Here's how the part is built. I have some questions about the finished solid (model axes, mm). Face numbers are marked on the shaded views. A direction names the side the tool comes from. Coordinates: 2 decimals unless noted, no trailing zeros. Write each loop counter-clockwise with the first axis right and the second up, starting at its lowest first coordinate (ties: lowest second). Pieces come first, ordered by that corner, then holes.
```python
from build123d import *

# Parameters (mm, degrees)
SKETCH1_R              = 2.35
PIN_DEPTH              = 11.35
SKETCH2_R              = 2.95
MIDDLE_DEPTH           = 4.8
SKETCH3_R              = 2.625
OUTER_RIM_DEPTH        = 0.5
BORE_CUT_DEPTH         = 13.562941535
SLOT_CUT_DEPTH         = 13.562941535
SLOT_CUT_DEPTH_BACK    = 13.562941535
SKETCH6_R              = 3.7
MIDDLE_BODY_DEPTH      = 3.9
MIDDLE_BORE_DEPTH      = 14.012398084
MIDDLE_BORE_DEPTH_BACK = 14.012398084
SKETCH7_R              = 2.4
SKETCH8_R              = 3.05
MIDDLE_RIM_CUT_DEPTH   = 0.75


with BuildPart() as part:
    # Sketch1 → Pin (new body)
    with BuildSketch(Plane(origin=(0, 0, 0), x_dir=(0, 0, -1), z_dir=(1, 0, 0))):
        Circle(SKETCH1_R)
    extrude(amount=PIN_DEPTH)

    # Sketch2 → Middle (add)
    with BuildSketch(Plane(origin=(0, 0, 0), x_dir=(0, 0, -1), z_dir=(1, 0, 0))):
        Circle(SKETCH2_R)
    extrude(amount=MIDDLE_DEPTH)

    # Sketch3 → Outer Rim (add)
    with BuildSketch(Plane(origin=(11.35, 0, 0), x_dir=(0, 0, -1), z_dir=(1, 0, 0))):
        Circle(SKETCH3_R)
    extrude(amount=OUTER_RIM_DEPTH)

    # Sketch4 → Bore Cut (cut, through all)
    with BuildSketch(Plane(origin=(0, 0, 0), x_dir=(0, 0, -1), z_dir=(1, 0, 0))):
        with BuildLine():
            ThreePointArc((-1.1, -1.393063172), (0, -1.775), (1.1, -1.393063172))
            Line((1.1, -1.393063172), (1.1, 1.393063172))
            ThreePointArc((1.1, 1.393063172), (0, 1.775), (-1.1, 1.393063172))
            Line((-1.1, 1.393063172), (-1.1, -1.393063172))
        make_face()
    extrude(amount=BORE_CUT_DEPTH, mode=Mode.SUBTRACT)

    # Sketch5 → Slot Cut (cut, two sides: drawn at the far end of the back side and taken through both)
    with BuildSketch(Plane.XY.offset(-SLOT_CUT_DEPTH_BACK)):
        with BuildLine():
            Line((14.3, -0.5), (9.4, -0.5))
            ThreePointArc((9.4, -0.5), (8.9, 0), (9.4, 0.5))
            Line((9.4, 0.5), (14.3, 0.5))
            ThreePointArc((14.3, 0.5), (14.8, 0), (14.3, -0.5))
        make_face()
        with BuildLine():
            Line((-14.3, -0.5), (-9.4, -0.5))
            ThreePointArc((-9.4, -0.5), (-8.9, 0), (-9.4, 0.5))
            Line((-9.4, 0.5), (-14.3, 0.5))
            ThreePointArc((-14.3, 0.5), (-14.8, 0), (-14.3, -0.5))
        make_face()
    extrude(amount=SLOT_CUT_DEPTH + SLOT_CUT_DEPTH_BACK, mode=Mode.SUBTRACT)

    # Sketch6 → Middle Body (add, symmetric)
    with BuildSketch(Plane.XY):
        Circle(SKETCH6_R)
    extrude(amount=MIDDLE_BODY_DEPTH, both=True)

    # Sketch7 → Middle Bore (cut, two sides: drawn at the far end of the back side and taken through both)
    with BuildSketch(Plane.XY.offset(-MIDDLE_BORE_DEPTH_BACK)):
        Circle(SKETCH7_R)
    extrude(amount=MIDDLE_BORE_DEPTH + MIDDLE_BORE_DEPTH_BACK, mode=Mode.SUBTRACT)

    # Sketch8 → Middle Rim Cut (cut)
    with BuildSketch(Plane.XY.offset(3.9)):
        Circle(SKETCH8_R)
    middle_rim_cut = extrude(amount=-MIDDLE_RIM_CUT_DEPTH, mode=Mode.SUBTRACT)

    # Mirror2: Middle Rim Cut across plane
    add(middle_rim_cut.mirror(Plane.XY), mode=Mode.SUBTRACT)


solid = part.part
```
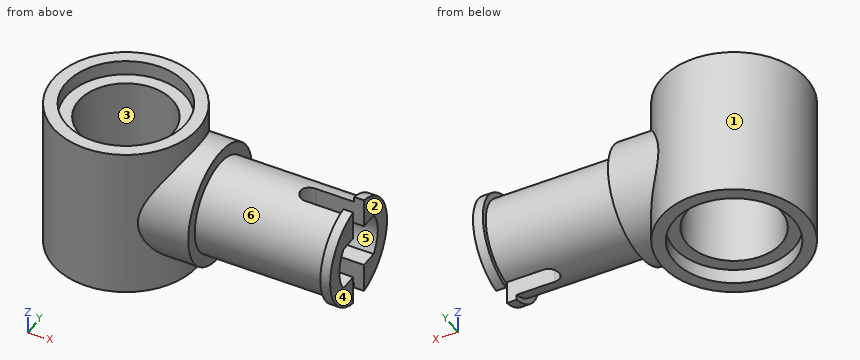
1) Will these pins go through, and if not, where does the flat tip stop? pin 1 (0.6 mm diameter, centred on y = 2, z = -0.5, fed in from -X); pin 2 (1.6 mm diameter, centred on x = 10.5, z = -1.5, fed in from +Y); pin 3 (1.6 mm diameter, centred on x = 11, z = -2, fed in from -Y).
Values follow:
pin 1: stops at x = -3.29
pin 2: stops at y = 2.24
pin 3: stops at y = -2.29
2) Imagine slicing it at D-D on z = 0. Please give me the cut outline in (x, y) (3 decimals).
Values follow:
outline: (2.233, -2.95) - (4.8, -2.95) - (4.8, -2.35) - (11.35, -2.35) - (11.35, -2.625) - (11.85, -2.625) - (11.85, -1.775) - (3.246, -1.775) arc R3.7 ccw to (3.246, 1.775) - (11.85, 1.775) - (11.85, 2.625) - (11.35, 2.625) - (11.35, 2.35) - (4.8, 2.35) - (4.8, 2.95) - (2.233, 2.95) arc R3.7 ccw (long way) to start; hole circle Ø4.8 at (0, 0)
3) We'd pull the mould along X, two halves only. Please class the marked faces 1, 2 and 3: pulls with the +X half, pulls with the -X half, needs draft (parallel to the pull), parting line crosses it, or undercut.
Values follow:
face 1: parting line crosses it
face 2: pulls with the +X half
face 3: undercut
4) Imagine slicing it at B-B on y = 0. Please give me the cut outline in (x, z).
Values follow:
outline: (-3.7, -3.9) - (-3.05, -3.9) - (-3.05, -3.15) - (-2.4, -3.15) - (-2.4, 3.15) - (-3.05, 3.15) - (-3.05, 3.9) - (-3.7, 3.9) - close; (2.4, -3.15) - (3.05, -3.15) - (3.05, -3.9) - (3.7, -3.9) - (3.7, -2.95) - (4.8, -2.95) - (4.8, -2.35) - (8.9, -2.35) - (8.9, -1.1) - (3.7, -1.1) - (3.7, 1.1) - (8.9, 1.1) - (8.9, 2.35) - (4.8, 2.35) - (4.8, 2.95) - (3.7, 2.95) - (3.7, 3.9) - (3.05, 3.9) - (3.05, 3.15) - (2.4, 3.15) - close
5) Imagine slicing it at A-A on x = 0. Please give me the cut outline in (y, z).
Values follow:
outline: (-3.7, -3.9) - (-3.05, -3.9) - (-3.05, -3.15) - (-2.4, -3.15) - (-2.4, 3.15) - (-3.05, 3.15) - (-3.05, 3.9) - (-3.7, 3.9) - close; (2.4, -3.15) - (3.05, -3.15) - (3.05, -3.9) - (3.7, -3.9) - (3.7, 3.9) - (3.05, 3.9) - (3.05, 3.15) - (2.4, 3.15) - close
6) On a 3-axis mill with a long thin cutter (end or side, diameter ignored), from which of +Z, -Z, +X, -X, +Y, -Y can I reach the whole of each face in a straight line? I mean the marked faces 4, 5 and 6. Say none if no direction works.
Values follow:
face 4: +Z, -Z, +X, +Y, -Y
face 5: +X
face 6: none
7) Imagine slicing it at C-C on x = 4. Please give me the cut outline in (y, z) (3 decimals).
Values follow:
outline: circle Ø5.9 at (0, 0); hole (-1.393, -1.1) - (1.393, -1.1) arc R1.775 ccw to (1.393, 1.1) - (-1.393, 1.1) arc R1.775 ccw to start
8) I need wall thicknesses on probe 1 along Y at (x, z) = (0, 0.25); probe 2 along Y at (x, z) = (0, -3.55); probe 3 along X at (y, z) = (1.5, -2). Which ranges of each line are inside material? Lowest first, please.
Values follow:
probe 1: y = -3.7 to -2.4, 2.4 to 3.7
probe 2: y = -3.7 to -3.05, 3.05 to 3.7
probe 3: x = -3.38 to -1.87, 1.87 to 4.8, 11.35 to 11.85
